from build123d import *

# Parameters (mm, degrees)
F0_W     = 355.6
F0_H     = 317.5
F1_DEPTH = 203.2
F3_SIZE2 = 304.8
F3_SIZE  = 88.9
F4_W     = 50.8
F4_H     = 317.5
F5_DEPTH = 558.8
F7_DEPTH = 12.7
F8_W     = 25.4
F8_H     = 292.1
F9_DEPTH = 12.7
F10_T    = -12.7
F13_R    = 7.62


with BuildPart() as f1:
    # F0 (on Front) → F1 (new body)
    with BuildSketch(Plane.XZ):
        Rectangle(F0_W, F0_H)
    extrude(amount=F1_DEPTH)

    # F3
    f3_edges = [f1.edges().sort_by_distance(p)[0] for p in [
        (0, -203.2, -158.75),
    ]]
    f3_side = f1.faces().sort_by_distance((0, -101.6, -158.75))[0]
    chamfer(f3_edges, length=F3_SIZE, length2=F3_SIZE2, reference=f3_side)

    # F4 (on face) → F5 (join)
    with BuildSketch(Plane(origin=(-177.8, 0, 0), x_dir=(0, -1, 0), z_dir=(-1, 0, 0))):
        with Locations((25.4, 0)):
            Rectangle(F4_W, F4_H)
    extrude(amount=F5_DEPTH)

    # F6 (on face) → F7 (cut)
    with BuildSketch(Plane.YZ.offset(177.8)):
        Polygon((-12.7, 146.05), (-189.9708333333, 146.05), (-104.775, -146.05), (-12.7, -146.05), align=None)
    extrude(amount=-F7_DEPTH, mode=Mode.SUBTRACT)

    # F8 (on face) → F9 (cut)
    with BuildSketch(Plane(origin=(-736.6, 0, 0), x_dir=(0, -1, 0), z_dir=(-1, 0, 0))):
        with Locations((25.4, 0)):
            Rectangle(F8_W, F8_H)
    extrude(amount=-F9_DEPTH, mode=Mode.SUBTRACT)

    # F10 (hollow: no face is removed)
    offset(amount=F10_T, kind=Kind.INTERSECTION, mode=Mode.SUBTRACT)

    # F13
    f13_edges = [f1.edges().sort_by_distance(p)[0] for p in [
        (-165.1, -38.1, 0),
    ]]
    fillet(f13_edges, radius=F13_R)


solid = f1.part
The model under review builds one solid part; all positions refer to its coordinate system, in mm. A direction names the side the tool comes from. Round coordinates to 2 decimals unless told otherwise and drop trailing zeros. Loops run counter-clockwise (first coordinate to the right, second up) from the corner with the lowest first, then second, coordinate; pieces in that order, holes last. Notation, with made-up numbers: M -4,-39 L 33,-39 A27 cw 33,-9 Z; hole C 39,41 d10. An arc over 180 degrees is marked long. Answer as CSV lines item,"result". Start each with the question number.
Item 1: Consider section A-A (y = -30). Write out the cut boundary in (x, z), then the cut area to 3 significant figures.
Item 2: Consider section D-D (y = -87). Write out the cut boundary in (x, z), then the cut area to 3 significant figures.
Item 3: For faces 1 (the face through (171.539, -147.969, 2.045)), 2 (the face through (-723.9, -25, 2)), 3 (the face through (177.8, -11, -1)), 4 (the face through (-177.4, -37.6, -146.05)), 5 (the face through (-453, -50.8, -2)), list the 3-axis set-ups (+Z, -Z, +X, -X, +Y, -Y) from which the entire face can be reached by the end or side of a thin tool; tool diameter is ignored.
Item 4: Insertion check: P1, Ø1.5, axis at y = -140.5, z = 119, coming from the +X side; P2, Ø10, axis at x = -733, z = -22, coming from the -Y side; P3, Ø1.5, axis at x = -163, z = 36.5, coming from the -Y side. Each pin has a flat end and moves straight along its axis. Give the tip position at first contact, or say it passes through.
Item 5: Consider section B-B (x = 47). Write out the cut boundary in (y, z) (3 decimals).
Item 6: Mouldability with a two-part tool opening along Z and no side actions: class faces 6 (the face through (-171, -44, -158.75)), 7 (the face through (-70, -78, 158.75)), 8 (the face through (165.1, -83, 2)), 9 (the face through (-736.6, -8, 2)) as released by +Z, released by -Z, zero draft, split by the parting line, or undercut.
Item 7: Wall thickness on line 1 (X direction, y = -113, z = -39); line 2 (X direction, y = -33, z = 72); line 3 (Y direction, x = -297, z = 100): over which ranges is each line inside the solid? List them lowest first. Write a range as [from, to].
Item 8: Consider section C-C (z = 19). Write out the cut boundary in (x, y), then the cut area to 3 significant figures.
Answer:
1,outline,"M -736.6,-158.75 L 177.8,-158.75 L 177.8,-146.05 L 165.1,-146.05 L 165.1,146.05 L 177.8,146.05 L 177.8,158.75 L -736.6,158.75 L -736.6,146.05 L -723.9,146.05 L -723.9,-146.05 L -736.6,-146.05 Z; hole M -711.2,-146.05 L 152.4,-146.05 L 152.4,146.05 L -711.2,146.05 Z"
1,area,"30,600 mm^2"
2,outline,"M -177.8,-158.75 L 177.8,-158.75 L 177.8,-146.05 L 165.1,-146.05 L 165.1,146.05 L 177.8,146.05 L 177.8,158.75 L -177.8,158.75 Z; hole M -165.1,-146.05 L 152.4,-146.05 L 152.4,146.05 L -165.1,146.05 Z"
2,area,"16,500 mm^2"
3,face 1,"+X"
3,face 2,"-X"
3,face 3,"+Z, -Z, +X, +Y, -Y"
3,face 4,"none"
3,face 5,"+Z, -Z, -X, -Y"
4,P1,"stops at x = 165.1"
4,P2,"stops at y = -50.8"
4,P3,"stops at y = -171.47"
5,outline,"M -203.2,146.05 L -114.3,-158.75 L 0,-158.75 L 0,158.75 L -203.2,158.75 Z; hole M -189.971,146.05 L -104.775,-146.05 L -12.7,-146.05 L -12.7,146.05 Z"
6,face 6,"released by -Z"
6,face 7,"released by +Z"
6,face 8,"undercut"
6,face 9,"zero draft"
7,line 1,"x = [-177.8, -165.1], [152.4, 165.1]"
7,line 2,"x = [-723.9, -711.2], [152.4, 165.1]"
7,line 3,"y = [-50.8, -38.1], [-12.7, 0]"
8,outline,"M -736.6,-50.8 L -177.8,-50.8 L -177.8,-166.14 L 177.8,-166.14 L 177.8,-152.91 L 165.1,-152.91 L 165.1,-12.7 L 177.8,-12.7 L 177.8,0 L -736.6,0 L -736.6,-12.7 L -723.9,-12.7 L -723.9,-38.1 L -736.6,-38.1 Z; hole M -711.2,-38.1 L -172.72,-38.1 A7.62 cw -165.1,-45.72 L -165.1,-152.91 L 152.4,-152.91 L 152.4,-12.7 L -711.2,-12.7 Z"
8,area,"27,000 mm^2"
